```python
from build123d import *

# Parameters (mm, degrees)
EXTRUDE_1_DEPTH = 70
SKETCH_2_W      = 10
SKETCH_2_H      = 8
EXTRUDE_2_DEPTH = 25
SKETCH_3_W      = 8
SKETCH_3_H      = 8
EXTRUDE_3_DEPTH = 10
SKETCH_5_R      = 1.6
EXTRUDE_4_DEPTH = 2.5
FILLET_1_R      = 2


with BuildPart() as part:
    # 草图1 → 凸台-拉伸1 (new body)
    with BuildSketch(Plane.XY):
        Polygon((0, -15), (10, 0), (-10, 0), align=None)
    extrude(amount=EXTRUDE_1_DEPTH)

    # 草图2 → 凸台-拉伸2 (add)
    with BuildSketch(Plane.XY):
        with Locations((0, 4)):
            Rectangle(SKETCH_2_W, SKETCH_2_H)
    extrude(amount=EXTRUDE_2_DEPTH)

    # 草图3 → 凸台-拉伸3 (add)
    with BuildSketch(Plane.XY.offset(70)):
        with Locations((0, 4)):
            Rectangle(SKETCH_3_W, SKETCH_3_H)
    extrude(amount=-EXTRUDE_3_DEPTH)

    # 草图5 → 凸台-拉伸4 (add, symmetric)
    with BuildSketch(Plane.XZ):
        with BuildLine():
            Line((-5.2, -2.5), (5.2, -2.5))
            ThreePointArc((5.2, -2.5), (9.979898987, -4.479898987), (8, 0.3))
            Line((8, 0.3), (-8, 0.3))
            ThreePointArc((-8, 0.3), (-9.979898987, -4.479898987), (-5.2, -2.5))
        make_face()
        with Locations((-8, -2.5)):
            Circle(SKETCH_5_R, mode=Mode.SUBTRACT)
        with Locations(Location((8, -2.5, 0), (0, 0, 180))):
            Circle(SKETCH_5_R, mode=Mode.SUBTRACT)
    extrude(amount=EXTRUDE_4_DEPTH, both=True)

    # 圆角1
    fillet_1_edges = [part.edges().sort_by_distance(p)[0] for p in [
        (0, -15, 35),
    ]]
    fillet(fillet_1_edges, radius=FILLET_1_R)


solid = part.part
```
Part model, mm, in its own coordinate system. A direction names the side the tool comes from. Round coordinates to 2 decimals unless told otherwise and drop trailing zeros. Write each loop counter-clockwise with the first axis right and the second up, starting at its lowest first coordinate (ties: lowest second). Pieces come first, ordered by that corner, then holes. Notation, with made-up numbers: M 43,32 L 81,32 A24 cw 81,42 Z; hole C 15,-31.5 d3. An arc over 180 degrees is marked long. Answer as CSV lines item,"result". Start each with the question number.
1) Which spindle directions (+Z, -Z, +X, -X, +Y, -Y) get a long thin tool onto all of the face, cutting with end or side? Do faces 4 (the face through (6, -6, 35)), 5 (the face through (-6, 1, 0.3)), 6 (the face through (4, 4, 65)), 7 (the face through (0, 5, 0)). Say none if no direction does.
2) Drill centre lines: L1, parallel to Z at x = 8, y = -0.95; L2, parallel to Z at x = 8, y = 0.7; L3, parallel to Z at x = 3.75, y = -0.25. Where is each one in solid material? Low to high.
3) Band-saw the part on B-B (x = 2.5). List the corners of the cut face in (y, z), then the cut area to 3 significant figures.
4) Drop flat-ended pins along their axis: pin 1 (0.6 mm diameter, centred on x = 9.5, y = -0.5, fed in from -Z); pin 2 (0.8 mm diameter, centred on x = 6, y = 1.5, fed in from +Z); pin 3 (8 mm diameter, centred on x = 4, y = 5, fed in from -Z). Give the stop position or say it passes through.
5) Mould opens along X. For faces 1 (the face through (0, 0, -2.5)), 2 (the face through (0.028, -13.394, 35.49)), 3 (the face through (0, -3, 70)) say: +X half, -X half, draft (parallel to the pull), parting line (faces both ways), or undercut.
6) Band-saw the part on C-C (y = -6). List the corners of the cut face in (x, z).
7) Band-saw the part on A-A (y = 4.5). List the corners of the cut face in (x, z).
8) Band-saw the part on D-D (z = 57). List the corners of the cut face in (x, y).
Worked out:
1,face 4,"+Z, +X, -Y"
1,face 5,"+Z, -X, +Y"
1,face 6,"+Z, +X, +Y"
1,face 7,"-Z, +X, -X, +Y"
2,L1,"-5.3 to -4.1, -0.9 to 70"
2,L2,"-5.3 to -4.1, -0.9 to 0.3"
2,L3,"-2.5 to 70"
3,outline,"M -11.25,0 L -2.5,0 L -2.5,-2.5 L 2.5,-2.5 L 2.5,0 L 8,0 L 8,25 L 0,25 L 0,60 L 8,60 L 8,70 L -11.25,70 Z"
3,area,"1,080 mm²"
4,pin 1,"z = -5.03"
4,pin 2,"z = 0.3"
4,pin 3,"z = -5.16"
5,face 1,"undercut"
5,face 2,"parting line"
5,face 3,"draft"
6,outline,"M -6,0 L 6,0 L 6,70 L -6,70 Z"
7,outline,"M -5,0 L 5,0 L 5,25 L -5,25 Z; M -4,60 L 4,60 L 4,70 L -4,70 Z"
8,outline,"M -10,0 L -1.66,-12.5 A2 ccw 1.66,-12.5 L 10,0 Z"
